from build123d import *

# Parameters (mm, degrees)
F0_R     = 1.75
F1_DEPTH = 2
F3_DEPTH = 2.5
F4_R     = 1.75
F5_DEPTH = 1.3


with BuildPart() as f1:
    # F0 (on Top) → F1 (new body)
    with BuildSketch(Plane.XY):
        with BuildLine():
            ThreePointArc((-13, -17), (-10.171573, -15.828427), (-9, -13))
            ThreePointArc((-9, -13), (-13, -9), (-17, -13))
            ThreePointArc((-17, -13), (-15.828427, -15.828427), (-13, -17))
        make_face()
        with Locations((-13, -13)):
            Circle(F0_R, mode=Mode.SUBTRACT)
        with BuildLine():
            ThreePointArc((-17, -13), (-13, -9), (-9, -13))
            ThreePointArc((-9, -13), (-10.171573, -15.828427), (-13, -17))
            Line((-13, -17), (13, -17))
            ThreePointArc((13, -17), (10.171573, -10.171573), (17, -13))
            Line((17, -13), (17, 13))
            ThreePointArc((17, 13), (10.171573, 10.171573), (13, 17))
            Line((13, 17), (-13, 17))
            ThreePointArc((-13, 17), (-10.171573, 15.828427), (-9, 13))
            ThreePointArc((-9, 13), (-13, 9), (-17, 13))
            Line((-17, 13), (-17, -13))
        make_face()
        with Locations((-7, -7)):
            Circle(F0_R, mode=Mode.SUBTRACT)
        with Locations((7, -7)):
            Circle(F0_R, mode=Mode.SUBTRACT)
        with Locations((-7, 7)):
            Circle(F0_R, mode=Mode.SUBTRACT)
        with Locations((7, 7)):
            Circle(F0_R, mode=Mode.SUBTRACT)
        with BuildLine():
            ThreePointArc((-13, 17), (-15.828427, 15.828427), (-17, 13))
            ThreePointArc((-17, 13), (-13, 9), (-9, 13))
            ThreePointArc((-9, 13), (-10.171573, 15.828427), (-13, 17))
        make_face()
        with Locations((-13, 13)):
            Circle(F0_R, mode=Mode.SUBTRACT)
        with BuildLine():
            ThreePointArc((17, -13), (10.171573, -10.171573), (13, -17))
            ThreePointArc((13, -17), (15.828427, -15.828427), (17, -13))
        make_face()
        with Locations((13, -13)):
            Circle(F0_R, mode=Mode.SUBTRACT)
        with BuildLine():
            ThreePointArc((17, 13), (15.828427, 15.828427), (13, 17))
            ThreePointArc((13, 17), (10.171573, 10.171573), (17, 13))
        make_face()
        with Locations((13, 13)):
            Circle(F0_R, mode=Mode.SUBTRACT)
    extrude(amount=F1_DEPTH)

    # F2 (on face) → F3 (join)
    with BuildSketch(Plane(origin=(0, 0, 0), x_dir=(1, 0, 0), z_dir=(0, 0, -1))):
        with BuildLine():
            ThreePointArc((-13, 17), (-15.828427, 15.828427), (-17, 13))
            Line((-17, 13), (-17, -13))
            ThreePointArc((-17, -13), (-15.828427, -15.828427), (-13, -17))
            Line((-13, -17), (13, -17))
            ThreePointArc((13, -17), (15.828427, -15.828427), (17, -13))
            Line((17, -13), (17, 13))
            ThreePointArc((17, 13), (15.828427, 15.828427), (13, 17))
            Line((13, 17), (-13, 17))
        make_face()
        Polygon((-11.25, -9.968911), (-9.5, -13), (-11.25, -16.031089), (-14.75, -16.031089), (-16.5, -13), (-14.75, -9.968911), align=None, mode=Mode.SUBTRACT)
        Polygon((-5.25, -3.968911), (-3.5, -7), (-5.25, -10.031089), (-8.75, -10.031089), (-10.5, -7), (-8.75, -3.968911), align=None, mode=Mode.SUBTRACT)
        Polygon((14.75, -9.968911), (16.5, -13), (14.75, -16.031089), (11.25, -16.031089), (9.5, -13), (11.25, -9.968911), align=None, mode=Mode.SUBTRACT)
        Polygon((8.75, -3.968911), (10.5, -7), (8.75, -10.031089), (5.25, -10.031089), (3.5, -7), (5.25, -3.968911), align=None, mode=Mode.SUBTRACT)
        Polygon((-8.75, 10.031089), (-5.25, 10.031089), (-3.5, 7), (-5.25, 3.968911), (-8.75, 3.968911), (-10.5, 7), align=None, mode=Mode.SUBTRACT)
        Polygon((-11.25, 16.031089), (-9.5, 13), (-11.25, 9.968911), (-14.75, 9.968911), (-16.5, 13), (-14.75, 16.031089), align=None, mode=Mode.SUBTRACT)
        Polygon((8.75, 10.031089), (10.5, 7), (8.75, 3.968911), (5.25, 3.968911), (3.5, 7), (5.25, 10.031089), align=None, mode=Mode.SUBTRACT)
        Polygon((11.25, 16.031089), (14.75, 16.031089), (16.5, 13), (14.75, 9.968911), (11.25, 9.968911), (9.5, 13), align=None, mode=Mode.SUBTRACT)
    extrude(amount=F3_DEPTH)

    # F4 (on face) → F5 (join)
    with BuildSketch(Plane.XY.offset(2)):
        with BuildLine():
            Line((-10.5, 10.5), (10.5, 10.5))
            Line((10.5, 10.5), (17, 10.5))
            Line((17, 10.5), (17, 13))
            ThreePointArc((17, 13), (15.828427, 15.828427), (13, 17))
            Line((13, 17), (-13, 17))
            ThreePointArc((-13, 17), (-15.828427, 15.828427), (-17, 13))
            Line((-17, 13), (-17, -13))
            ThreePointArc((-17, -13), (-15.828427, -15.828427), (-13, -17))
            Line((-13, -17), (13, -17))
            ThreePointArc((13, -17), (15.828427, -15.828427), (17, -13))
            Line((17, -13), (17, -10.5))
            Line((17, -10.5), (10.5, -10.5))
            Line((10.5, -10.5), (-10.5, -10.5))
            Line((-10.5, -10.5), (-10.5, 10.5))
        make_face()
        with Locations((-13, -13)):
            Circle(F4_R, mode=Mode.SUBTRACT)
        with Locations((13, -13)):
            Circle(F4_R, mode=Mode.SUBTRACT)
        with Locations((-13, 13)):
            Circle(F4_R, mode=Mode.SUBTRACT)
        with Locations((13, 13)):
            Circle(F4_R, mode=Mode.SUBTRACT)
    extrude(amount=F5_DEPTH)


solid = f1.part
Input: part model. Units: mm. Frame: model coordinates. A direction names the side the tool comes from. Coordinates: 2 decimals unless noted, no trailing zeros. Order: outer loops, then holes, each group sorted by start corner. A loop starts at its lowest first (then second) coordinate and runs counter-clockwise, first axis right, second up. Notation, with made-up numbers: M 86.25,39 L 115.25,39 A22 cw 115.25,47 Z; hole C -12,22.25 d7. An arc over 180 degrees is marked long. Write item = value, one per line. Start each with the question number.
(1) Section B-B on z = 1.25. Give the number of separate pieces and of enclosed holes in the cut face, and give its area (3 significant figures).
(2) Pull-direction query (Y, two-part tool) for faces 1 (the flat face through (-10.36, 14.49, -1.23)), 2 (the flat face through (-17, 0, 0)), 3 (the cylindrical face through (-15.797, 15.859, 0.359)); classes: released by +Y, released by -Y, zero draft, split by the parting line, or undercut.
(3) Reachability of faces 4 (the flat face through (9.64, -5.51, -1.23)), 5 (the flat face through (3, 10.5, 3)), 6 (the cylindrical face through (-13.228, -11.265, 1.627)) from +Z, -Z, +X, -X, +Y, -Y: full face, straight path, thin tool, end or side. Return the list, or none.
(4) First-contact query: P1, Ø3, axis at x = 7, y = 7, coming from the -Z side; P2, Ø3, axis at x = -12, y = -12.5, coming from the -Z side; P3, Ø6, axis at x = 8, y = 3.5, coming from the +Z side. Flat tips, straight axial feed; report the tip coordinate or a pass-through.
(5) Section A-A on x = 7. Output: boundary loops of the cut face in (y, z).
(6) Section C-C on y = 12.5. Output: boundary loops of the cut face in (x, z).
(7) Section D-D on x = -2. Output: boundary loops of the cut face in (y, z), and give its area (3 significant figures).
(8) Line query: line 1 along Y through (x, z) = (-13, 0.95); line 2 along Y through (x, z) = (-7, 1.4); line 3 along X through (y, z) = (-7, -0.1). Output: solid intervals per line, ascending. Write a range as [from, to].
Result set:
q1.separate_pieces = 1
q1.enclosed_holes = 8
q1.area = 1,070 mm²
q2.face_1 = undercut
q2.face_2 = zero draft
q2.face_3 = released by +Y
q3.face_4 = -Z
q3.face_5 = +Z, +X
q3.face_6 = +Z, -Z
q4.P1 = through
q4.P2 = 0
q4.P3 = 2
q5.outline = M -17,-2.5 L -10.03,-2.5 L -10.03,0 L -8.75,0 L -8.75,2 L -10.5,2 L -10.5,3.3 L -17,3.3 Z; M -5.25,0 L -3.97,0 L -3.97,-2.5 L 3.97,-2.5 L 3.97,0 L 5.25,0 L 5.25,2 L -5.25,2 Z; M 8.75,0 L 10.03,0 L 10.03,-2.5 L 17,-2.5 L 17,3.3 L 10.5,3.3 L 10.5,2 L 8.75,2 Z
q6.outline = M -17,-2.5 L -16.21,-2.5 L -16.21,0 L -14.68,0 L -14.68,3.3 L -17,3.3 Z; M -11.32,0 L -9.79,0 L -9.79,-2.5 L 9.79,-2.5 L 9.79,0 L 11.32,0 L 11.32,3.3 L -11.32,3.3 Z; M 14.68,0 L 16.21,0 L 16.21,-2.5 L 17,-2.5 L 17,3.3 L 14.68,3.3 Z
q7.outline = M -17,-2.5 L 17,-2.5 L 17,3.3 L 10.5,3.3 L 10.5,2 L -10.5,2 L -10.5,3.3 L -17,3.3 Z
q7.area = 170 mm²
q8.line_1 = [-17, -14.75], [-11.25, 11.25], [14.75, 17]
q8.line_2 = [-17, -8.75], [-5.25, 5.25], [8.75, 17]
q8.line_3 = [-17, -10.5], [-3.5, 3.5], [10.5, 17]
